Print and shaded views of the part. All mm, measured from the part's lowest x, y and z. A direction names the side the tool comes from. Give positions to 0.01 mm unless a question says otherwise; leave off trailing zeros. Loops run counter-clockwise (first coordinate to the right, second up) from the corner with the lowest first, then second, coordinate; pieces in that order, holes last. Notation, with made-up numbers: M 75,66 L 123,66 A21 ccw 123,104 Z; hole C -11.5,89.25 d5. An arc over 180 degrees is marked long. Answer in a Markdown table with one row per item.
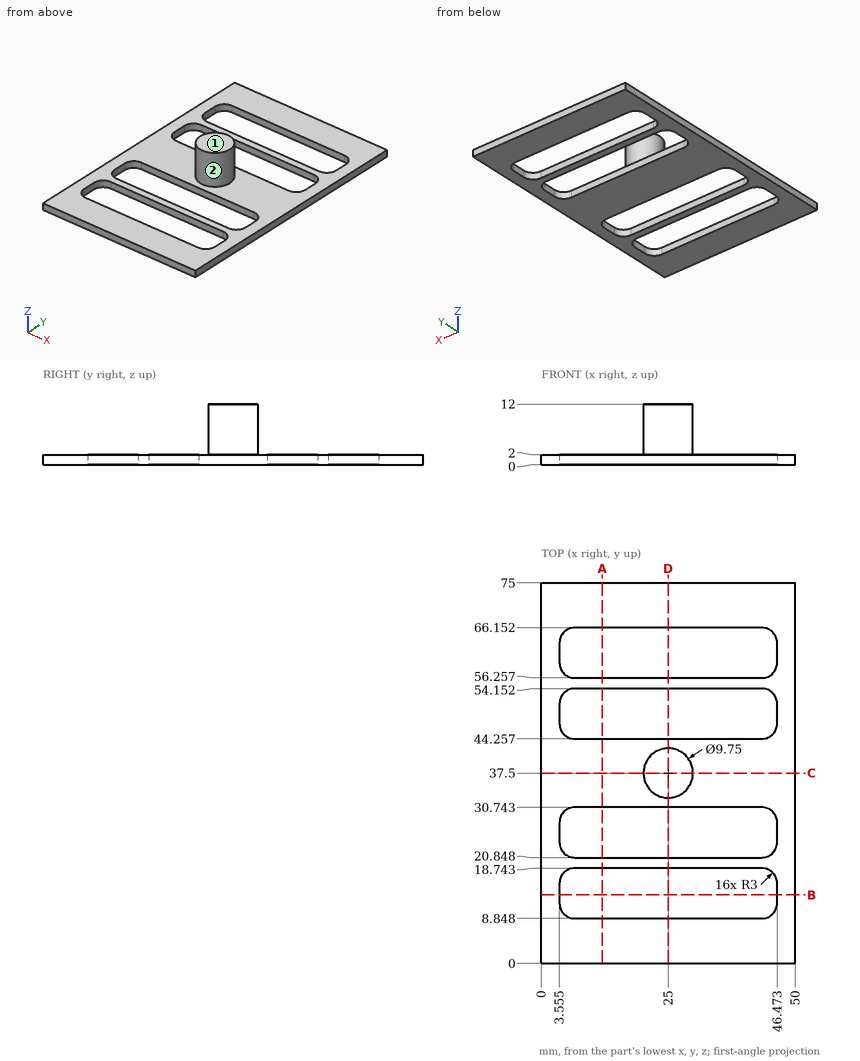
(1) Saw through at B-B, the plane y = 13.5. Give the cut face in (x, z) (1 decimal).
Established:
| item | result |
|---|---|
| outline | M 0,0 L 3.6,0 L 3.6,2 L 0,2 Z; M 46.5,0 L 50,0 L 50,2 L 46.5,2 Z |
(2) Saw through at C-C, the plane y = 37.5. Give the cut face in (x, z) (1 decimal).
Established:
| item | result |
|---|---|
| outline | M 0,0 L 50,0 L 50,2 L 29.9,2 L 29.9,12 L 20.1,12 L 20.1,2 L 0,2 Z |
(3) Wall check: L1, parallel to Y at x = 14, z = 1.25; L2, parallel to Z at x = 4, y = 57.5; L3, parallel to Y at x = 23.5, z = 6. Give the ranges that are in metal, low to high.
Established:
| item | result |
|---|---|
| L1 | y = 0 to 8.85, 18.74 to 20.85, 30.74 to 44.26, 54.15 to 56.26, 66.15 to 75 |
| L2 | z = 0 to 2 |
| L3 | y = 32.86 to 42.14 |
(4) Saw through at A-A, the plane x = 12. Give the cut face in (y, z).
Established:
| item | result |
|---|---|
| outline | M 0,0 L 8.85,0 L 8.85,2 L 0,2 Z; M 18.74,0 L 20.85,0 L 20.85,2 L 18.74,2 Z; M 30.74,0 L 44.26,0 L 44.26,2 L 30.74,2 Z; M 54.15,0 L 56.26,0 L 56.26,2 L 54.15,2 Z; M 66.15,0 L 75,0 L 75,2 L 66.15,2 Z |
(5) Flat gauge pins, fed straight in: P1, Ø1, axis at x = 32.5, y = 40, coming from the +Z side; P2, Ø1.5, axis at x = 41.5, z = 4.5, coming from the +Y side. Where does each tip first touch, or does it go through?
Established:
| item | result |
|---|---|
| P1 | stops at z = 2 |
| P2 | passes through |
(6) Saw through at D-D, the plane x = 25. Give the cut face in (y, z) (1 decimal), and give its area (3 significant figures).
Established:
| item | result |
|---|---|
| outline | M 0,0 L 8.8,0 L 8.8,2 L 0,2 Z; M 18.7,0 L 20.8,0 L 20.8,2 L 18.7,2 Z; M 30.7,0 L 44.3,0 L 44.3,2 L 42.4,2 L 42.4,12 L 32.6,12 L 32.6,2 L 30.7,2 Z; M 54.2,0 L 56.3,0 L 56.3,2 L 54.2,2 Z; M 66.2,0 L 75,0 L 75,2 L 66.2,2 Z |
| area | 168 mm2 |
(7) Which spindle directions (+Z, -Z, +X, -X, +Y, -Y) get a long thin tool onto all of the face, cutting with end or side? Do the marked faces 1 and 2. Say none if no direction does.
Established:
| item | result |
|---|---|
| face 1 | +Z, +X, -X, +Y, -Y |
| face 2 | +Z |
